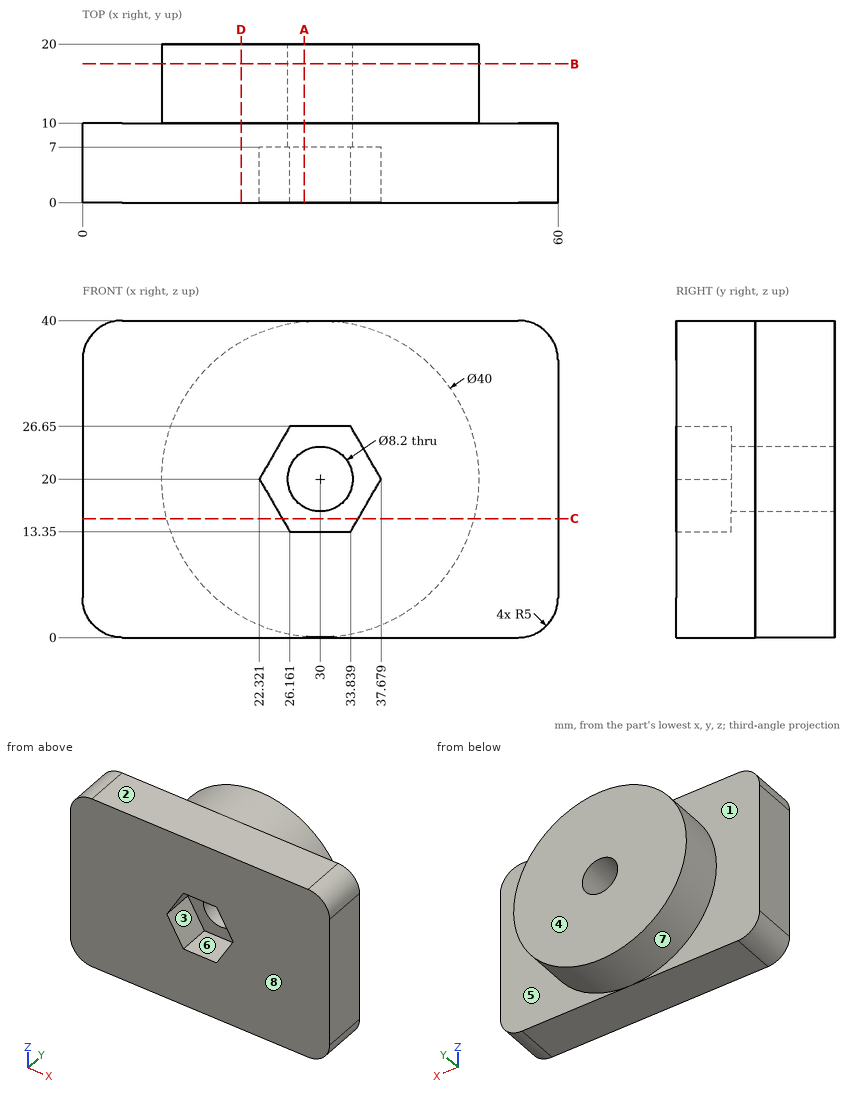
Study the drawing (mm; zero at the part's minimum x, y, z) and answer. A direction names the side the tool comes from. Give positions to 0.01 mm unless a question says otherwise; leave off trailing zeros. Write each loop counter-clockwise with the first axis right and the second up, starting at its lowest first coordinate (ties: lowest second). Pieces come first, ordered by that corner, then holes. Notation, with made-up numbers: (38, 85.25) - (95, 85.25) arc R34 ccw to (95, 117.25) - close; hole circle Ø10 at (-5, 83). An arc over 180 degrees is marked (long way). Use a Markdown table: item, result.
1. Find the intervals of material crossed by probe 1 along X at (y, z) = (16.75, 20); probe 2 along Y at (x, z) = (6, 27); probe 3 along Y at (x, z) = (25.5, 21.5), in increasing order. Write a range as from..to.
Values follow:
| item | result |
|---|---|
| probe 1 | x = 10..25.9, 34.1..50 |
| probe 2 | y = 0..10 |
| probe 3 | y = 7..20 |
2. For a pull along Z with two mould halves and no side action, classify the marked faces 1, 2 and 3 as released by +Z, released by -Z, zero draft, split by the parting line, or undercut.
Values follow:
| item | result |
|---|---|
| face 1 | zero draft |
| face 2 | released by +Z |
| face 3 | undercut |
3. Section B-B on y = 17.5 is taken. Write down the section's boundary in (x, z).
Values follow:
| item | result |
|---|---|
| outline | circle Ø40 at (30, 20); hole circle Ø8.2 at (30, 20) |
4. Section A-A on x = 28 is taken. Write down the section's boundary in (y, z).
Values follow:
| item | result |
|---|---|
| outline | (0, 0) - (10, 0) - (10, 0.1) - (20, 0.1) - (20, 16.42) - (7, 16.42) - (7, 13.35) - (0, 13.35) - close; (0, 26.65) - (7, 26.65) - (7, 23.58) - (20, 23.58) - (20, 39.9) - (10, 39.9) - (10, 40) - (0, 40) - close |
5. Section C-C on z = 15 is taken. Write down the section's boundary in (x, y) (1 decimal), plus the area to 3 significant figures.
Values follow:
| item | result |
|---|---|
| outline | (0, 0) - (25.2, 0) - (25.2, 7) - (34.8, 7) - (34.8, 0) - (60, 0) - (60, 10) - (49.4, 10) - (49.4, 20) - (10.6, 20) - (10.6, 10) - (0, 10) - close |
| area | 920 mm² |
6. Each of these flat-tipped pins is pushed along its axis until it touches: P1, Ø4, axis at x = 27.5, y = 12.5, coming from the -Z side; P2, Ø6.5, axis at x = 32.5, z = 19.5, coming from the -Y side. Where does it stop, or does it pass through?
Values follow:
| item | result |
|---|---|
| P1 | stops at z = 0.01 |
| P2 | stops at y = 7 |
7. A tool of negligible diameter and unlimited length cuts with its end or side. For the marked faces 4, 5, 6, 7 and 8, from which of +Z, -Z, +X, -X, +Y, -Y can it reach the whole face along a straight path? Write none if from no direction.
Values follow:
| item | result |
|---|---|
| face 4 | +Z, -Z, +X, -X, +Y |
| face 5 | +X, +Y |
| face 6 | -Y |
| face 7 | +Y |
| face 8 | +Z, -Z, +X, -X, -Y |
8. Section D-D on x = 20 is taken. Write down the section's boundary in (y, z).
Values follow:
| item | result |
|---|---|
| outline | (0, 0) - (10, 0) - (10, 2.68) - (20, 2.68) - (20, 37.32) - (10, 37.32) - (10, 40) - (0, 40) - close |
